Read the model definition and answer for the solid it produces. Units are mm, in the model's axes. A direction names the side the tool comes from. Round coordinates to 2 decimals unless told otherwise and drop trailing zeros. Loops run counter-clockwise (first coordinate to the right, second up) from the corner with the lowest first, then second, coordinate; pieces in that order, holes last. Notation, with made-up numbers: (28, 55.25) - (44, 55.25) arc R19 ccw to (44, 87.25) - close; hole circle Ø5 at (-26.75, 19). An arc over 180 degrees is marked (long way). Answer as CSV lines item,"result".
```python
from build123d import *

# Parameters (mm, degrees)
SKETCH_1_R               = 1.75
EXTRUDE_1_DEPTH          = 3
EXTRUDE_2_DEPTH          = 11
EXTRUDE_2_DEPTH_BACK     = 3
CUT_EXTRUDE_1_DEPTH      = 79.296095621
CUT_EXTRUDE_1_DEPTH_BACK = 79.296095621
SKETCH_4_R               = 75.737398045
SKETCH_4_R_2             = 60
FILLET_1_R               = 1


with BuildPart() as part:
    # Эскиз1 → Бобышка-Вытянуть1 (new body)
    with BuildSketch(Plane(origin=(0, 0, 0), x_dir=(1, 0, 0), z_dir=(0, 1, 0))):
        with BuildLine():
            Line((15.39090645, 42.286167935), (17.785047453, 48.864016281))
            ThreePointArc((17.785047453, 48.864016281), (23.097425832, 46.588720952), (28.124517408, 43.737987157))
            ThreePointArc((28.124517408, 43.737987157), (32.887215772, 48.124766732), (39.210044191, 46.72871103))
            ThreePointArc((39.210044191, 46.72871103), (52.827549631, 30.5), (60.073272934, 10.592538838))
            ThreePointArc((60.073272934, 10.592538838), (60.118729466, 8.455730047), (59.51728837, 6.404806668))
            Line((59.51728837, 6.404806668), (54.192372599, -4.949615977))
            Line((54.192372599, -4.949615977), (44.777960949, 4.464774712))
            ThreePointArc((44.777960949, 4.464774712), (35.534315772, 27.610005481), (15.39090645, 42.286167935))
        make_face()
        with Locations(Location((34.710530923, 41.366399928, 0), (0, 0, 270))):
            Circle(SKETCH_1_R, mode=Mode.SUBTRACT)
        with Locations(Location((46.765371804, 27, 0), (0, 0, 270))):
            Circle(SKETCH_1_R, mode=Mode.SUBTRACT)
        with Locations(Location((53.179618663, 9.377001594, 0), (0, 0, 270))):
            Circle(SKETCH_1_R, mode=Mode.SUBTRACT)
    extrude(amount=EXTRUDE_1_DEPTH)

    # Эскиз2 → Бобышка-Вытянуть2 (add, two sides: drawn at the far end of the back side and taken through both)
    with BuildSketch(Plane(origin=(0, 3, 0), x_dir=(1, 0, 0), z_dir=(0, 1, 0)).offset(-EXTRUDE_2_DEPTH_BACK)):
        with BuildLine():
            Line((52.071067812, -7.071067812), (52.071067812, -5.656854249))
            Line((52.071067812, -5.656854249), (50.656854249, -5.656854249))
            Line((50.656854249, -5.656854249), (50.656854249, -4.242640687))
            Line((50.656854249, -4.242640687), (49.242640687, -4.242640687))
            Line((49.242640687, -4.242640687), (49.242640687, -2.828427125))
            Line((49.242640687, -2.828427125), (47.828427125, -2.828427125))
            Line((47.828427125, -2.828427125), (47.828427125, -1.414213562))
            Line((47.828427125, -1.414213562), (46.414213562, -1.414213562))
            Line((46.414213562, -1.414213562), (46.414213562, 0))
            Line((46.414213562, 0), (45, 0))
            ThreePointArc((45, 0), (36.861841993, 25.810939636), (15.39090645, 42.286167935))
            Line((15.39090645, 42.286167935), (16.41696688, 45.105245798))
            ThreePointArc((16.41696688, 45.105245798), (38.518692264, 28.641060494), (47.922027533, 2.734826717))
            Line((47.922027533, 2.734826717), (54.899494937, -4.242640687))
            Line((54.899494937, -4.242640687), (52.071067812, -7.071067812))
        make_face()
    extrude(amount=EXTRUDE_2_DEPTH + EXTRUDE_2_DEPTH_BACK)

    # Эскиз4 → Вырез-Вытянуть1 (cut, two sides: drawn at the far end of the back side and taken through both)
    with BuildSketch(Plane(origin=(0, 3, 0), x_dir=(1, 0, 0), z_dir=(0, 1, 0)).offset(-CUT_EXTRUDE_1_DEPTH_BACK)):
        Circle(SKETCH_4_R)
        Circle(SKETCH_4_R_2, mode=Mode.SUBTRACT)
    extrude(amount=CUT_EXTRUDE_1_DEPTH + CUT_EXTRUDE_1_DEPTH_BACK, mode=Mode.SUBTRACT)

    # Скругление1
    # the kernel refuses this fillet: 1 mm, written as the material it adds along each edge
    with BuildSketch(Plane(origin=(54.643826402, 0, 3.986972152), x_dir=(0.7071067811866617, 0, 0.7071067811864333), z_dir=(0, 1, 0))) as fillet_1_piece_1:
        with BuildLine():
            CenterArc((0.726813354, 0.93091204), FILLET_1_R, 199.874698522, 48.702735989)
            Line((-0.213624991, 0.590947748), (-0.232433757, 0.584148463))
            Line((-0.232433757, 0.584148463), (-0.018808767, -0.006799286))
            Line((-0.018808767, -0.006799286), (0, -0.02))
            ThreePointArc((0, -0.02), (0.180784955, -0.02), (0.35426504, -0.018618241))
            Line((0.35426504, -0.018618241), (0.361569909, 0))
        make_face()
    extrude(amount=3)


solid = part.part
```
1) A cutting plane is placed at B-B, the plane y = 8.75. Determine the outline of the cut face in (x, z), plus the area to 3 significant figures.
Entries:
outline,"(15.39, -42.29) - (16.42, -45.11) arc R48 ccw to (47.92, -2.73) - (54.9, 4.24) - (52.07, 7.07) - (52.07, 5.66) - (50.66, 5.66) - (50.66, 4.24) - (49.24, 4.24) - (49.24, 2.83) - (47.83, 2.83) - (47.83, 1.41) - (46.41, 1.41) - (46.41, 0) - (45, 0) arc R45 cw to start"
area,"201 mm^2"
2) Each of these flat-tipped pins is pushed along its axis until it touches: P1, Ø12, axis at x = 43, z = -42.5, coming from the +Y side; P2, Ø1.5, axis at y = 11, z = -25, coming from the +X side; P3, Ø1.6, axis at y = 9, z = 5, coming from the -X side. Where does it stop, or does it pass through?
Entries:
P1,"stops at y = 3"
P2,"stops at x = 41.42"
P3,"stops at x = 49.24"
3) A cutting plane is placed at D-D, the plane z = -34. Determine the outline of the cut face in (x, y).
Entries:
outline,"(29.48, 0) - (49.44, 0) - (49.44, 3) - (33.88, 3) - (33.88, 14) - (29.48, 14) - close"
4) A cutting plane is placed at C-C, the plane x = 42.5. Determine the outline of the cut face in (y, z), plus the area to 3 significant figures.
Entries:
outline,"(0, -42.35) - (3, -42.35) - (3, -22.31) - (14, -22.31) - (14, -14.79) - (0, -14.79) - close"
area,"165 mm^2"
5) The mould has two halves that part along X. Classify faces 1 (the face through (50, 7, 4.243)), 2 (the face through (47.828, 7, 2)), 3 (the face through (51.627, 1.479, -8.569)): pulls with the +X half, pulls with the -X half, needs draft (parallel to the pull), parting line crosses it, or undercut.
Entries:
face 1,"needs draft"
face 2,"pulls with the -X half"
face 3,"undercut"
6) A cutting plane is placed at A-A, the plane z = -27. Determine the outline of the cut face in (x, y), plus the area to 3 significant figures.
Entries:
outline,"(36, 0) - (45.02, 0) - (45.02, 3) - (39.69, 3) - (39.69, 14) - (36, 14) - close; (48.52, 0) - (53.58, 0) - (53.58, 3) - (48.52, 3) - close"
area,"82.8 mm^2"
7) A tool of negligible diameter and unlimited length cuts with its end or side. For faces 4 (the face through (51, 7, 5.657)), 5 (the face through (38.284, 8.423, -28.954)), 6 (the face through (34.787, 1.479, -43.115)), from which of +Z, -Z, +X, -X, +Y, -Y can it reach the whole face along a straight path? Write none if from no direction.
Entries:
face 4,"+Z, -X, +Y, -Y"
face 5,"-Z, +X, +Y"
face 6,"+Y, -Y"
8) Find the intervals of material crossed by line 1 (Y direction, x = 41, z = -28); line 2 (Z direction, x = 46.5, y = 1.5); line 3 (X direction, y = 2.2, z = -27), in increasing order.
Entries:
line 1,"y = 0 to 3"
line 2,"z = -37.92 to -28.73, -25.27 to 1.41"
line 3,"x = 36 to 45.02, 48.52 to 53.58"
